Model file for the job. Use its own axes, mm. A direction names the side the tool comes from. Coordinates: 2 decimals unless noted, no trailing zeros. Order: outer loops, then holes, each group sorted by start corner. A loop starts at its lowest first (then second) coordinate and runs counter-clockwise, first axis right, second up. Notation, with made-up numbers: M 38.25,60.5 L 86.25,60.5 A27 cw 86.25,94.5 Z; hole C 61,64.25 d9. An arc over 180 degrees is marked long. Return JSON: item names as keys, results as strings.
```python
from build123d import *

# Parameters (mm, degrees)
F0_W     = 914.4
F0_H     = 1828.8
F1_DEPTH = 152.4
F2_W     = 914.4
F2_H     = 152.4
F2_H_2   = 914.4
F3_DEPTH = 152.4
F7_W     = 88.9
F7_H     = 1306.8192187859
F8_DEPTH = 88.9


with BuildPart() as f1:
    # F0 (on Front) → F1 (new body)
    with BuildSketch(Plane.XZ):
        with Locations((-457.2, 914.4)):
            Rectangle(F0_W, F0_H)
    extrude(amount=F1_DEPTH)

    # F2 (on Top) → F3 (join)
    with BuildSketch(Plane.XY):
        with Locations((-457.2, -76.2)):
            Rectangle(F2_W, F2_H)
        with Locations((-457.2, -609.6)):
            Rectangle(F2_W, F2_H_2)
    extrude(amount=-F3_DEPTH)

    # F7 (on 3pt) → F8 (join)
    with BuildSketch(Plane(origin=(0, -784.4117647059, 470.6470588235), x_dir=(-1, 0, 0), z_dir=(0, 0.8574929257, -0.5144957554))):
        Polygon((435.5678258105, -548.8640718901), (524.4678258105, -548.8640718901), (524.4678258105, -503.1253992326), (524.4678258105, -78.4091531272), (435.5678258105, -78.4091531272), (435.5678258105, -503.1253992326), align=None)
        with Locations((480.0178258105, 575.0004562658)):
            Rectangle(F7_W, F7_H)
    extrude(amount=F8_DEPTH)


solid = f1.part
```
Item 1: Saw through at A-A (z = 184). Write the cut outline in (x, y).
Check result:
{"outline": "M -914.4,-152.4 L 0,-152.4 L 0,0 L -914.4,0 Z; M -524.47,-956.4 L -435.57,-956.4 L -435.57,-852.73 L -524.47,-852.73 Z"}
Item 2: Wall check: line 1 (Y direction, x = -396, z = 1278.5). Give the ranges that are in metal, low to high.
Check result:
{"line 1": "y = -152.4 to 0"}
Item 3: Saw through at C-C (y = -400.5). Write the cut outline in (x, z), and give its area (3 significant figures).
Check result:
{"outline": "M -914.4,-152.4 L 0,-152.4 L 0,0 L -914.4,0 Z; M -524.47,937.71 L -435.57,937.71 L -435.57,1110.5 L -524.47,1110.5 Z", "area": "155,000 mm2"}
Item 4: Saw through at B-B (x = -504). Write the cut outline in (y, z), and give its area (3 significant figures).
Check result:
{"outline": "M -1066.8,-152.4 L 0,-152.4 L 0,1828.8 L -152.4,1828.8 L -152.4,1524 L -1066.8,0 Z; hole M -963.13,0 L -152.4,0 L -152.4,1351.21 Z", "area": "590,000 mm2"}
Item 5: 3-axis set-ups, long thin cutter, end or side, ignore diameter. For faces 1 (the flat face through (-464, -75, 1828.8)), 2 (the flat face through (-524.468, -578, 729)): which of +Z, -Z, +X, -X, +Y, -Y reach the whole face in a straight line?
Check result:
{"face 1": "+Z, +X, -X, +Y, -Y", "face 2": "+Z, -X, -Y"}
Item 6: Drop flat-ended pins along their axis: pin 1 Ø12 at (y, z) = (-423.5, 908.5) entering from +X; pin 2 Ø3 at (x, y) = (-206.5, -913) entering from +Z; pin 3 Ø4 at (x, z) = (-607, 1463) entering from -Y. Give the stop position or say it passes through.
Check result:
{"pin 1": "stops at x = -435.57", "pin 2": "stops at z = 0", "pin 3": "stops at y = -152.4"}
Item 7: Pull direction Z, two halves, no side cores. Call faces 3 (the flat face through (-479.4, -552.09, 685.06)), 4 (the flat face through (-464, -526, -152.4)), 5 (the flat face through (-435.568, -566, 750)): +Z half, -Z half, draft (parallel to the pull), parting line (faces both ways), or undercut.
Check result:
{"face 3": "undercut", "face 4": "-Z half", "face 5": "draft"}
Item 8: Saw through at D-D (z = 1441.5). Write the cut outline in (x, y).
Check result:
{"outline": "M -914.4,-152.4 L -524.47,-152.4 L -524.47,-201.9 L -435.57,-201.9 L -435.57,-152.4 L 0,-152.4 L 0,0 L -914.4,0 Z"}
